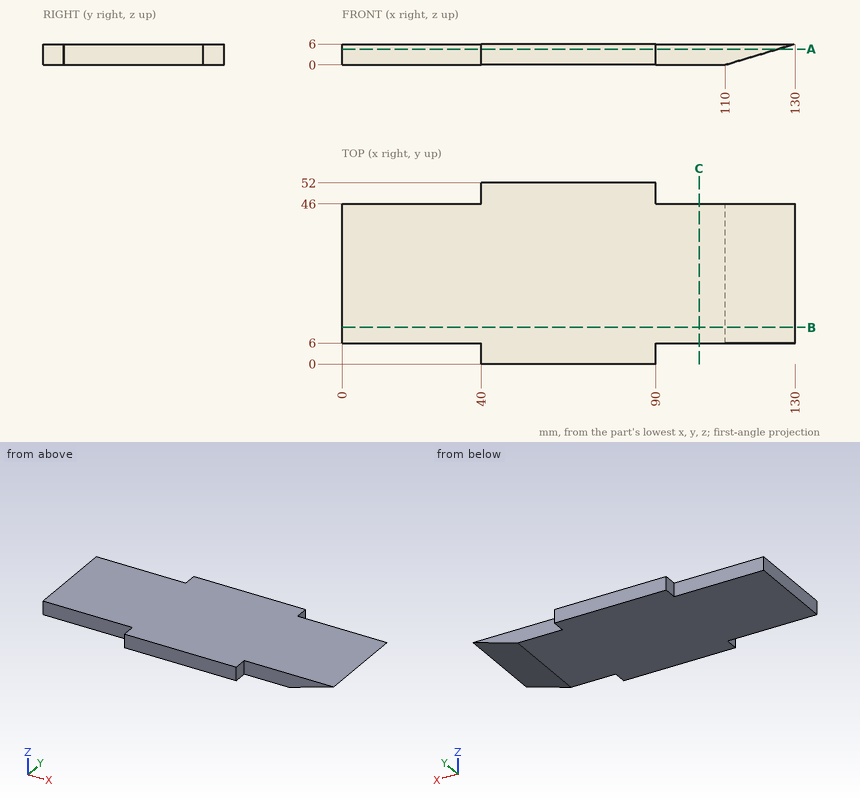
Can you work these out from the drawing? Everything is in mm from the part's minimum corner. Round coordinates to 2 decimals unless told otherwise and drop trailing zeros. Loops run counter-clockwise (first coordinate to the right, second up) from the corner with the lowest first, then second, coordinate; pieces in that order, holes last.
1. For P1, Ø3, axis at y = 2, z = 2, coming from the -X side; P2, Ø1.8, axis at y = 2, z = 3, coming from the +X side; P3, Ø3, axis at x = 25, z = 4, coming from the +Y side, each with a flat end and sliding along its axis, tell me the tip position at first contact or that it passes through.
Answer list:
P1: stops at x = 40
P2: stops at x = 90
P3: stops at y = 46
2. If we section it at B-B on y = 10.5: Write out the boundary of the cut face in (x, z), plus the area to 3 significant figures.
Answer list:
outline: (0, 0) - (110, 0) - (130, 6) - (0, 6) - close
area: 720 mm2
3. If I drill on line 1 along X through (y, z) = (4.5, 2.5); line 2 along Y through (x, z) = (11, 2.25), over which ranges is the centre line in solid material (lowest first)?
Answer list:
line 1: x = 40 to 90
line 2: y = 6 to 46
4. If we section it at C-C on x = 102.5: Write out the boundary of the cut face in (y, z), plus the area to 3 significant figures.
Answer list:
outline: (6, 0) - (46, 0) - (46, 6) - (6, 6) - close
area: 240 mm2
5. If we section it at A-A on z = 4.5: Write out the boundary of the cut face in (x, y).
Answer list:
outline: (0, 6) - (40, 6) - (40, 0) - (90, 0) - (90, 6) - (125, 6) - (125, 46) - (90, 46) - (90, 52) - (40, 52) - (40, 46) - (0, 46) - close
